Autodesk Inventor part; units mm, degrees
ref_plane "YZ Plane" through (0, 0, 0) normal (1, 0, 0) x (0, 1, 0)
ref_plane "XZ Plane" through (0, 0, 0) normal (0, 1, 0) x (-1, 0, 0)
ref_plane "XY Plane" through (0, 0, 0) normal (0, 0, 1) x (1, 0, 0)
sketch "Sketch1" plane through (0, 0, 0) normal (0, 0, 1) x (1, 0, 0)
  line L0 (-62, -15.65) -> (62, -15.65)
  line L1 (62, -15.65) -> (62, 15.65)
  line L2 (62, 15.65) -> (-62, 15.65)
  line L3 (-62, 15.65) -> (-62, -15.65)
  line L4 (-62, -15.65) -> (62, 15.65) construction
  line L5 (62, -15.65) -> (-62, 15.65) construction
  line L6 (-62, 0) -> (62, 0) construction
  line L7 (-46.35, -15.65) -> (46.35, -15.65)
  line L8 (46.35, 15.65) -> (-46.35, 15.65)
  arc A0 (-46.35, 15.65) -> (-46.35, -15.65) centre (-46.35, 0) ccw
  arc A1 (46.35, -15.65) -> (46.35, 15.65) centre (46.35, 0) ccw
  point P0 (0, 0)
  point P1 (0, 0)
  point P2 (-62, 0)
  point P3 (-46.35, 15.65)
  point P4 (62, 0)
  point P5 (46.35, -15.65)
  dimension "d0" = 124
  dimension "d1" = 31.3
extrude "Extrusion1" add sketch "Sketch1" along normal blind 24.5
sketch "Sketch2" plane through (0, 0, 24.5) normal (0, 0, 1) x (1, 0, 0)
  circle A0 centre (0, 0) radius 11.975
  circle A1 centre (0, 0) radius 7.8185
  dimension "d4" = 23.95
extrude "Extrusion2" add sketch "Sketch2" along normal blind 2.25
chamfer "Chamfer1" distance 3.175 angle 85 1 edges at (62, 0, 24.5) measured on face at (62, -5.2167, 8.1667)
chamfer "Chamfer2" distance 3.175 angle 85 1 edges at (-62, 0, 24.5) measured on face at (-62, 5.2167, 8.1667)
extrude "Extrusion3" cut sketch "Sketch1" along normal blind 24.5 contours L3 A0 L0 | L3 L2 A0 | A1 L1 L0 | A1 L2 L1
chamfer "Chamfer3" distance 2 angle 45 2 edges at (62, 0, 0) (-62, 0, 0)
sketch "Sketch4" plane through (0, 0, 0) normal (1, 0, 0) x (0, 1, 0)
  line L0 (15.65, 24.5) -> (-15.65, 24.5) construction
  line L1 (-15.65, 24.5) -> (-15.65, 0) construction
  line L2 (-15.65, 10.6) -> (-24.65, 10.6)
  line L3 (-24.65, 10.6) -> (-24.65, 18.35)
  line L4 (-24.65, 18.35) -> (-15.65, 18.35)
  line L5 (-15.65, 18.35) -> (-15.65, 10.6)
  circle A0 centre (-20.5, 14.475) radius 2.25
  arc A1 (-21.9856, 18.35) -> (-21.9856, 10.6) centre (-20.5, 14.475) ccw
  line L6 (-15.65, 14.475) -> (-24.65, 14.475) construction
  point P0 (0, 0)
  point P1 (-13.65, 0)
  point P2 (-15.65, 2)
  dimension "d19" = 10.6
  dimension "d20" = 9
  dimension "d21" = 7.75
  dimension "d22" = 4.5
  dimension "d23" = 1.9
extrude "Extrusion4" add sketch "Sketch4" along normal mid plane 20.2 contours L2 A1 L4 L5
properties part number "Emeet_Camera"
Geometry check sheet. Reference: the model listing, model coordinates, mm. A direction names the side the tool comes from. Coordinates: 2 decimals unless noted, no trailing zeros. Order: outer loops, then holes, each group sorted by start corner. A loop starts at its lowest first (then second) coordinate and runs counter-clockwise, first axis right, second up. Notation, with made-up numbers: M -10.75,-34 L 0.25,-34 A29 ccw 0.25,-11 Z; hole C 64.25,-12 d8. An arc over 180 degrees is marked long. Answer as a JSON object with one key per item and string values.
Q1. Cross-section at C-C on z = 9.25. Record the cut outline in (x, y), and give its area (3 significant figures).
Results are:
{"outline": "M -46.35,-15.65 L 46.35,-15.65 A15.65 ccw 46.35,15.65 L -46.35,15.65 A15.65 ccw Z", "area": "3,670 mm²"}
Q2. Release check for a two-part mould opening along X. For faces 1 (the flat face through (-12, 4, 24.5)), 2 (the flat face through (43.601, 0.219, 22.935)), 3 (the flat face through (-43.601, -0.219, 22.935)), 4 (the flat face through (0, 0, 24.5)) record: released by +X, released by -X, zero draft, split by the parting line, or undercut.
Results are:
{"face 1": "zero draft", "face 2": "released by +X", "face 3": "released by -X", "face 4": "undercut"}
Q3. Scan lines: line 1 (Y direction, x = 0, z = 26.05) (1 decimal); line 2 (Z direction, x = 1.75, y = -20.5) (3 decimals); line 3 (Y direction, x = 4, z = 10.5). Record each from-to range of solid material in increasing order.
Results are:
{"line 1": "y = -12 to -7.8, 7.8 to 12", "line 2": "z = 10.6 to 12.225, 16.725 to 18.35", "line 3": "y = -15.65 to 15.65"}
Q4. Depth check by flat-ended pin: pin 1 Ø1.5 at (y, z) = (3.5, 21) entering from +X; pin 2 Ø7 at (x, y) = (0, -17.5) entering from -Z; pin 3 Ø4 at (y, z) = (-20.5, 15.5) entering from -X; pin 4 Ø3.5 at (y, z) = (-20.5, 14.475) entering from -X. Enter the tip coordinate at first touch or a pass-through.
Results are:
{"pin 1": "stops at x = 61.76", "pin 2": "stops at z = 0.35", "pin 3": "stops at x = -10.1", "pin 4": "passes through"}
Q5. Cross-section at D-D on x = -29.5. Record the cut outline in (y, z), and give its area (3 significant figures).
Results are:
{"outline": "M -15.65,2 L -13.65,0 L 13.65,0 L 15.65,2 L 15.65,24.17 L -15.65,24.17 Z", "area": "752 mm²"}
Q6. Tool access check on faces 5 (the flat face through (0, -19, 10.6)), 6 (the cylindrical face through (-2.6, 11.69, 25.61)), 7 (the flat face through (10.1, -18, 15)). Record the directions out of +Z, -Z, +X, -X, +Y, -Y that give a thin tool (end or side, any length) a straight path to the whole face; none if there is none.
Results are:
{"face 5": "-Z, +X, -X, -Y", "face 6": "+Z", "face 7": "+Z, -Z, +X, -Y"}
Q7. Cross-section at A-A on y = -20.5. Record the cut outline in (x, z) (3 decimals), and give its area (4 significant figures).
Results are:
{"outline": "M -10.1,10.6 L 10.1,10.6 L 10.1,12.225 L -10.1,12.225 Z; M -10.1,16.725 L 10.1,16.725 L 10.1,18.35 L -10.1,18.35 Z", "area": "65.65 mm²"}
Q8. Cross-section at B-B on x = -2.5. Record the cut outline in (y, z) (3 decimals), and give its area (3 significant figures).
Results are:
{"outline": "M -21.986,10.6 L -15.65,10.6 L -15.65,2 L -13.65,0 L 13.65,0 L 15.65,2 L 15.65,24.5 L 11.711,24.5 L 11.711,26.75 L 7.408,26.75 L 7.408,24.5 L -7.408,24.5 L -7.408,26.75 L -11.711,26.75 L -11.711,24.5 L -15.65,24.5 L -15.65,18.35 L -21.986,18.35 A4.15 ccw Z; hole C -20.5,14.475 d4.5", "area": "830 mm²"}
